from build123d import *

# Parameters (mm, degrees)
SKICA1_W                = 300
SKICA1_H                = 300
P_IDAT_VYSUNUT_M1_DEPTH = 10
P_IDAT_VYSUNUT_M3_DEPTH = 10


with BuildPart() as part:
    # Skica1 → Přidat vysunutím1 (new body)
    with BuildSketch(Plane.XY):
        with Locations((150, 150)):
            Rectangle(SKICA1_W, SKICA1_H)
    extrude(amount=P_IDAT_VYSUNUT_M1_DEPTH)

    # Skica3 → Přidat vysunutím3 (add)
    with BuildSketch(Plane.XY.offset(10)):
        with BuildLine():
            Line((121.527137935, 14.364823185), (134.527137935, 14.364823185))
            Line((134.527137935, 14.364823185), (134.527137935, 57))
            Line((134.527137935, 57), (149.527137935, 42))
            Line((149.527137935, 42), (194.472862065, 42))
            Line((194.472862065, 42), (209.472862065, 57))
            Line((209.472862065, 57), (209.472862065, 14.364823185))
            Line((209.472862065, 14.364823185), (222.472862065, 14.364823185))
            Line((222.472862065, 14.364823185), (248.153836395, 75.999073478))
            ThreePointArc((248.153836395, 75.999073478), (251.029031296, 85.424046933), (252, 95.22986613))
            Line((252, 95.22986613), (252, 110))
            ThreePointArc((252, 110), (172, 190), (92, 110))
            Line((92, 110), (92, 95.22986613))
            ThreePointArc((92, 95.22986613), (92.970968704, 85.424046933), (95.846163605, 75.999073478))
            Line((95.846163605, 75.999073478), (121.527137935, 14.364823185))
        make_face()
        with BuildLine():
            ThreePointArc((131, 82.99166898), (106.532275896, 106.185322904), (139.47140521, 99))
            Line((139.47140521, 99), (204.52859479, 99))
            ThreePointArc((204.52859479, 99), (222.500204374, 115.492849842), (239.5, 98))
            ThreePointArc((239.5, 98), (230.624094155, 82.772557667), (213, 82.99166898))
            Line((213, 82.99166898), (191, 58))
            Line((191, 58), (179, 58))
            Line((179, 58), (179, 84))
            Line((179, 84), (165, 84))
            Line((165, 84), (165, 58))
            Line((165, 58), (153, 58))
            Line((153, 58), (131, 82.99166898))
        make_face(mode=Mode.SUBTRACT)
    extrude(amount=P_IDAT_VYSUNUT_M3_DEPTH)


solid = part.part
Work out the finished part from the listing and answer in its coordinate system (mm). A direction names the side the tool comes from. Round coordinates to 2 decimals unless told otherwise and drop trailing zeros. Write each loop counter-clockwise with the first axis right and the second up, starting at its lowest first coordinate (ties: lowest second). Pieces come first, ordered by that corner, then holes. Notation, with made-up numbers: (60, 84) - (102, 84) arc R19 cw to (102, 117) - close; hole circle Ø9 at (76, 13.25). An arc over 180 degrees is marked (long way). Answer in a Markdown table with one row per item. Add a question column.
1. The mould has two halves that part along Y. Classify faces 1 (the flat face through (159, 58, 15)), 2 (the flat face through (115, 185, 10)), 3 (the flat face through (148, 0, 5)): +Y half, -Y half, draft (parallel to the pull), parting line (faces both ways), or undercut.
2. A cutting plane is placed at A-A, the plane z = 15.75. Determine the outline of the cut face in (x, y), and give its area (3 significant figures).
3. Find the intervals of material crossed by line 1 along X through (y, z) = (98, 17); line 2 along Z through (x, y) = (144, 205); line 3 along Y through (x, z) = (182, 17.75), in increasing order. Write a range as from..to.
4. A cutting plane is placed at B-B, the plane x = 172. Determine the outline of the cut face in (y, z), and give its area (3 significant figures).
5. A cutting plane is placed at D-D, the plane x = 41. Determine the outline of the cut face in (y, z), and give its area (3 significant figures).
6. Given pin 1 (8 mm diameter, centred on y = 69.5, z = 14.5, fed in from +X); pin 2 (2 mm diameter, centred on x = 61.5, z = 12.5, fed in from -Y); pin 3 (5 mm diameter, centred on y = 103, z = 13.5, fed in from +X); pin 4 (3 mm diameter, centred on x = 156, z = 14.5, fed in from +Y), each flat-ended and moving along its own axis, determine where each tip first touches the part or whether it passes through.
7. For faces 4 (the flat face through (216, 14.365, 15)), 5 (the cylindrical face through (251, 85.29, 14.93)), 6 (the flat face through (185, 58, 15)), 7 (the cylindrical face through (92.944, 85.56, 14.93)), 8 (the flat face through (92, 103, 15)), determine the directions among +Z, -Z, +X, -X, +Y, -Y from which every point of the face is accessible in a straight line to the end or side of a thin tool.
8. A cutting plane is placed at C-C, the plane y = 173.5. Determine the outline of the cut face in (x, z).
Worked out:
| question | item | result |
|---|---|---|
| 1 | face 1 | undercut |
| 1 | face 2 | draft |
| 1 | face 3 | -Y half |
| 2 | outline | (92, 95.23) arc R50 ccw to (95.85, 76) - (121.53, 14.36) - (134.53, 14.36) - (134.53, 57) - (149.53, 42) - (194.47, 42) - (209.47, 57) - (209.47, 14.36) - (222.47, 14.36) - (248.15, 76) arc R50 ccw to (252, 95.23) - (252, 110) arc R80 ccw to (92, 110) - close; hole (131, 82.99) - (153, 58) - (165, 58) - (165, 84) - (179, 84) - (179, 58) - (191, 58) - (213, 82.99) arc R17.5 ccw (long way) to (204.53, 99) - (139.47, 99) arc R17.5 ccw (long way) to start |
| 2 | area | 16,800 mm^2 |
| 3 | line 1 | 92..104.5, 239.5..252 |
| 3 | line 2 | 0..10 |
| 3 | line 3 | 42..58, 99..189.37 |
| 4 | outline | (0, 0) - (300, 0) - (300, 10) - (190, 10) - (190, 20) - (99, 20) - (99, 10) - (84, 10) - (84, 20) - (42, 20) - (42, 10) - (0, 10) - close |
| 4 | area | 4,330 mm^2 |
| 5 | outline | (0, 0) - (300, 0) - (300, 10) - (0, 10) - close |
| 5 | area | 3,000 mm^2 |
| 6 | pin 1 | x = 247.11 |
| 6 | pin 2 | through |
| 6 | pin 3 | x = 252 |
| 6 | pin 4 | y = 188.67 |
| 7 | face 4 | +Z, +X, -X, -Y |
| 7 | face 5 | +Z, +X, -Y |
| 7 | face 6 | +Z |
| 7 | face 7 | +Z, -X, -Y |
| 7 | face 8 | +Z, -X, +Y, -Y |
| 8 | outline | (0, 0) - (300, 0) - (300, 10) - (220.66, 10) - (220.66, 20) - (123.34, 20) - (123.34, 10) - (0, 10) - close |
